```python
from build123d import *

# Parameters (mm, degrees)
SKETCH_1_R                      = 8.5
EXTRUDE_1_DEPTH                 = 20
SKETCH_2_R                      = 3.2
CUT_EXTRUDE_1_DEPTH             = 9
CUT_EXTRUDE_2_REACH             = 25.335
SKETCH_3_R                      = 1
CUT_EXTRUDE_2_DIRECTION_2_REACH = 25.335
CUT_EXTRUDE_3_DEPTH             = 21
CUT_EXTRUDE_3_DEPTH_BACK        = 19
SKETCH_4_R                      = 1
SKETCH_5_R                      = 2
CUT_EXTRUDE_4_DEPTH             = 8
CUT_EXTRUDE_6_DEPTH             = 3.2
SKETCH_10_W                     = 3.2
SKETCH_10_H                     = 8.08
CUT_EXTRUDE_8_DEPTH             = 7.75


with BuildPart() as part:
    # 草图1 → 凸台-拉伸1 (new body)
    with BuildSketch(Plane(origin=(0, 0, 0), x_dir=(0, 0, -1), z_dir=(1, 0, 0))):
        Circle(SKETCH_1_R)
    extrude(amount=EXTRUDE_1_DEPTH)

    # 草图2 → 切除-拉伸1 (cut)
    with BuildSketch(Plane.ZY):
        Circle(SKETCH_2_R)
    extrude(amount=-CUT_EXTRUDE_1_DEPTH, mode=Mode.SUBTRACT)

    # 草图3 → 切除-拉伸2 (cut, up to next)
    with BuildSketch(Plane(origin=(0, 0, 0), x_dir=(1, 0, 0), z_dir=(0, 1, 0)), mode=Mode.PRIVATE) as cut_extrude_2_sk1:
        with Locations(Location((3, 0, 0), (0, 0, 270))):
            Circle(SKETCH_3_R)
    cut_extrude_2_tool1 = extrude(cut_extrude_2_sk1.sketch, amount=-CUT_EXTRUDE_2_REACH, mode=Mode.PRIVATE) & part.part
    add(cut_extrude_2_tool1.solids().sort_by_distance((3, 0, 0))[0], mode=Mode.SUBTRACT)

    # 草图3 → 切除-拉伸2 direction 2 (cut, up to next)
    with BuildSketch(Plane(origin=(0, 0, 0), x_dir=(1, 0, 0), z_dir=(0, 1, 0)), mode=Mode.PRIVATE) as cut_extrude_2_direction_2_sk1:
        with Locations(Location((3, 0, 0), (0, 0, 270))):
            Circle(SKETCH_3_R)
    cut_extrude_2_direction_2_tool1 = extrude(cut_extrude_2_direction_2_sk1.sketch, amount=CUT_EXTRUDE_2_DIRECTION_2_REACH, mode=Mode.PRIVATE) & part.part
    add(cut_extrude_2_direction_2_tool1.solids().sort_by_distance((3, 0, 0))[0], mode=Mode.SUBTRACT)

    # 草图4 → 切除-拉伸3 (cut, two sides: drawn at the far end of the back side and taken through both)
    with BuildSketch(Plane.XY.offset(-CUT_EXTRUDE_3_DEPTH_BACK)):
        with Locations(Location((6, 0, 0), (0, 0, 180))):
            Circle(SKETCH_4_R)
    extrude(amount=CUT_EXTRUDE_3_DEPTH + CUT_EXTRUDE_3_DEPTH_BACK, mode=Mode.SUBTRACT)

    # 草图5 → 切除-拉伸4 (cut)
    with BuildSketch(Plane(origin=(20, 0, 0), x_dir=(0, 0, -1), z_dir=(1, 0, 0))):
        with Locations((0, 4.25)):
            Circle(SKETCH_5_R)
        with Locations((0, -4.25)):
            Circle(SKETCH_5_R)
    extrude(amount=-CUT_EXTRUDE_4_DEPTH, mode=Mode.SUBTRACT)

    # 草图8 → 切除-拉伸6 (cut)
    with BuildSketch(Plane(origin=(18, 0, 0), x_dir=(0, 0, -1), z_dir=(1, 0, 0))):
        Polygon((-4.041451884, 4.25), (-2.020725942, 0.75), (2.020725942, 0.75), (4.041451884, 4.25), (2.020725942, 7.75), (-2.020725942, 7.75), align=None)
        Polygon((4.041451884, -4.25), (2.020725942, -0.75), (-2.020725942, -0.75), (-4.041451884, -4.25), (-2.020725942, -7.75), (2.020725942, -7.75), align=None)
    extrude(amount=-CUT_EXTRUDE_6_DEPTH, mode=Mode.SUBTRACT)

    # 草图10 → 切除-拉伸8 (cut)
    with BuildSketch(Plane(origin=(0, 8.5, 0), x_dir=(1, 0, 0), z_dir=(0, 1, 0))):
        with Locations((16.4, 0)):
            Rectangle(SKETCH_10_W, SKETCH_10_H)
    cut_extrude_8 = extrude(amount=-CUT_EXTRUDE_8_DEPTH, mode=Mode.SUBTRACT)

    # 镜向1: 切除-拉伸8 across plane
    add(cut_extrude_8.mirror(Plane.ZX), mode=Mode.SUBTRACT)


solid = part.part
```
For this review, take the finished solid that the model builds, in its own axes (mm). A direction names the side the tool comes from. Coordinates: 2 decimals unless noted, no trailing zeros. Write each loop counter-clockwise with the first axis right and the second up, starting at its lowest first coordinate (ties: lowest second). Pieces come first, ordered by that corner, then holes. Notation, with made-up numbers: (9, -38) - (48, -38) arc R19 cw to (48, -29) - close; hole circle Ø1 at (77, -34.75). An arc over 180 degrees is marked (long way). Answer in a Markdown table with one row per item. Add a question column.
Q1. For P1, Ø5, axis at x = 8.5, y = 3, coming from the +Z side; P2, Ø3.5, axis at y = 4.25, z = 0, coming from the +X side; P3, Ø1, axis at x = 16, y = 6.5, coming from the -Z side; P4, Ø1.2, axis at x = 3, z = 0, coming from the -Y side, all flat-tipped, find the tip position at first contact; note any pin that passes through.
Q2. Draft analysis for pull direction X (two halves, no side actions). For faces 4 (the flat face through (16, 6, 4.04)), 5 (the cylindrical face through (19.014, -6.202, 0.434)), 6 (the flat face through (12, -4, 0)), state which applies: +X half, -X half, draft (parallel to the pull), parting line (faces both ways), or undercut.
Q3. We need section A-A, the plane y = 0. State the section outline as (x, z) points, and give its area (3 significant figures).
Q4. We need section B-B, the plane z = 0. Count the separate pieces of the cut face and the enclosed holes in it, and give its area (3 significant figures).
Q5. For probe 1 along X at (y, z) = (-6.75, 0); probe 2 along Y at (x, z) = (12.65, 0); probe 3 along X at (y, z) = (-7.25, -0.5), list the stretches that pass through material, from the lowest coordinate up.
Q6. Tool access review of faces 1 (the flat face through (16, -3, 4.04)), 2 (the flat face through (16, 3, 4.04)), 3 (the cylindrical face through (4.437, 0.961, 3.052)): name each direction out of +Z, -Z, +X, -X, +Y, -Y from which nothing blocks a thin tool from reaching the whole face with its end or side.
Q7. We need section D-D, the plane y = 3.75. State the section outline as (x, z) points.
Answer list:
| question | item | result |
|---|---|---|
| 1 | P1 | stops at z = 8.49 |
| 1 | P2 | stops at x = 12 |
| 1 | P3 | stops at z = -6.02 |
| 1 | P4 | passes through |
| 2 | face 4 | undercut |
| 2 | face 5 | draft |
| 2 | face 6 | +X half |
| 3 | outline | (0, -8.5) - (5, -8.5) - (5, -3.2) - (0, -3.2) - close; (0, 3.2) - (5, 3.2) - (5, 8.5) - (0, 8.5) - close; (7, -8.5) - (20, -8.5) - (20, 8.5) - (7, 8.5) - (7, 3.2) - (9, 3.2) - (9, -3.2) - (7, -3.2) - close |
| 3 | area | 261 mm2 |
| 4 | separate pieces | 5 |
| 4 | enclosed holes | 0 |
| 4 | area | 173 mm2 |
| 5 | probe 1 | x = 0 to 2, 4 to 14.8, 18 to 20 |
| 5 | probe 2 | y = -8.5 to -6.25, -2.25 to 2.25, 6.25 to 8.5 |
| 5 | probe 3 | x = 0 to 2.13, 3.87 to 14.8, 18 to 20 |
| 6 | face 1 | -Y |
| 6 | face 2 | +Y |
| 6 | face 3 | -X |
| 7 | outline | (0, -7.63) - (20, -7.63) - (20, -1.94) - (18, -1.94) - (18, -4.04) - (14.8, -4.04) - (14.8, -1.94) - (12, -1.94) - (12, 1.94) - (14.8, 1.94) - (14.8, 4.04) - (18, 4.04) - (18, 1.94) - (20, 1.94) - (20, 7.63) - (0, 7.63) - close; hole circle Ø2 at (3, 0) |
